Check sheet for the modelled part. Datum: model origin and axes. Units: mm. A direction names the side the tool comes from. Coordinates: 2 decimals unless noted, no trailing zeros. Order: outer loops, then holes, each group sorted by start corner. A loop starts at its lowest first (then second) coordinate and runs counter-clockwise, first axis right, second up. Notation, with made-up numbers: (-20.5, 29) -> (-1.5, 29) arc R30 cw to (-1.5, 68) -> close; hole circle Ø3 at (34.25, 34.25). An arc over 180 degrees is marked (long way). Put each result on its own line as item: value. Start each with the question number.
```python
from build123d import *

# Parameters (mm, degrees)
SKETCH1_W           = 98
SKETCH1_H           = 25
BOSS_EXTRUDE1_DEPTH = 10
CUT_EXTRUDE4_DEPTH  = 10
SKETCH4_W           = 25
SKETCH4_H           = 10
CUT_EXTRUDE6_DEPTH  = 5
SKETCH5_W           = 25
SKETCH5_H           = 10
CUT_EXTRUDE7_DEPTH  = 5
SKETCH6_W           = 5
SKETCH6_H           = 10
CUT_EXTRUDE8_DEPTH  = 5
SKETCH7_W           = 5
SKETCH7_H           = 10
CUT_EXTRUDE9_DEPTH  = 5
SKETCH8_W           = 88
SKETCH8_H           = 5
CUT_EXTRUDE10_DEPTH = 2


with BuildPart() as part:
    # Sketch1 → Boss-Extrude1 (new body)
    with BuildSketch(Plane(origin=(0, 0, 0), x_dir=(1, 0, 0), z_dir=(0, 1, 0))):
        Rectangle(SKETCH1_W, SKETCH1_H)
    extrude(amount=BOSS_EXTRUDE1_DEPTH)

    # Sketch2 → Cut-Extrude4 (cut)
    with BuildSketch(Plane(origin=(0, 10, 0), x_dir=(1, 0, 0), z_dir=(0, 1, 0))):
        Polygon((-2.5, 2.403992328), (-2.5, -7.5), (-34, -7.5), (-34, 7.5), (-2.5, 7.5), align=None)
        Polygon((2.5, 2.403992328), (2.5, 7.5), (34, 7.5), (34, -7.5), (2.5, -7.5), align=None)
    extrude(amount=-CUT_EXTRUDE4_DEPTH, mode=Mode.SUBTRACT)

    # Sketch4 → Cut-Extrude6 (cut)
    with BuildSketch(Plane.ZY.offset(49)):
        with Locations((0, 5)):
            Rectangle(SKETCH4_W, SKETCH4_H)
    extrude(amount=-CUT_EXTRUDE6_DEPTH, mode=Mode.SUBTRACT)

    # Sketch5 → Cut-Extrude7 (cut)
    with BuildSketch(Plane(origin=(49, 0, 0), x_dir=(0, 0, -1), z_dir=(1, 0, 0))):
        with Locations((0, 5)):
            Rectangle(SKETCH5_W, SKETCH5_H)
    extrude(amount=-CUT_EXTRUDE7_DEPTH, mode=Mode.SUBTRACT)

    # Sketch6 → Cut-Extrude8 (cut)
    with BuildSketch(Plane(origin=(44, 0, 0), x_dir=(0, 0, -1), z_dir=(1, 0, 0))):
        with Locations((0, 5)):
            Rectangle(SKETCH6_W, SKETCH6_H)
    extrude(amount=-CUT_EXTRUDE8_DEPTH, mode=Mode.SUBTRACT)

    # Sketch7 → Cut-Extrude9 (cut)
    with BuildSketch(Plane.ZY.offset(44)):
        with Locations((0, 5)):
            Rectangle(SKETCH7_W, SKETCH7_H)
    extrude(amount=-CUT_EXTRUDE9_DEPTH, mode=Mode.SUBTRACT)

    # Sketch8 → Cut-Extrude10 (cut)
    with BuildSketch(Plane(origin=(0, 0, -12.5), x_dir=(-1, 0, 0), z_dir=(0, 0, -1))):
        with Locations((0, 7.5)):
            Rectangle(SKETCH8_W, SKETCH8_H)
    extrude(amount=-CUT_EXTRUDE10_DEPTH, mode=Mode.SUBTRACT)


solid = part.part
```
1) Sectioned sample at C-C (x = 22). Record the boundary of the cut face in (y, z), plus the area to 3 significant figures.
2) Scan lines: line 1 along X through (y, z) = (8.75, -7); line 2 along X through (y, z) = (3.5, 1.5); line 3 along Z through (x, y) = (-29.5, 3). Record each from-to range of solid material in increasing order. Write a range as [from, to].
3) Access from +Z, -Z, +X, -X, +Y, -Y to the whole of each face (thin tool, end or side, straight path). Record for faces 3 (the flat face through (-39, 5, 0)), 4 (the flat face through (1, 5, -12)), 5 (the flat face through (42, 5, -2.5)), 6 (the flat face through (-1, 0, 0)), 7 (the flat face through (34, 5, 0)).
4) Sectioned sample at D-D (z = -0.5). Record the boundary of the cut face in (x, y).
5) Sectioned sample at A-A (z = 4). Record the boundary of the cut face in (x, y).
6) Gauge pin test, flat ends, axial feed: pin 1 (1 mm diameter, centred on x = -7.5, z = -11.5, fed in from +Y); pin 2 (12 mm diameter, centred on x = 11.5, z = 5, fed in from +Y); pin 3 (2.5 mm diameter, centred on y = 6.5, z = -1, fed in from +X); pin 4 (8 mm diameter, centred on x = 25.5, z = 0.5, fed in from +Y). Record the tip position at first contact, or that the pin passes through.
7) Sectioned sample at B-B (y = 7.75). Record the boundary of the cut face in (x, z), plus the area to 3 significant figures.
8) Mould release check, pull along Z, two halves, no side actions. Record for faces 1 (the flat face through (-44, 5, 7)), 2 (the flat face through (-2.5, 5, 0)): +Z half, -Z half, draft (parallel to the pull), parting line (faces both ways), or undercut.
Entries:
1. outline: (0, -12.5) -> (5, -12.5) -> (5, -10.5) -> (10, -10.5) -> (10, -7.5) -> (0, -7.5) -> close; (0, 7.5) -> (10, 7.5) -> (10, 12.5) -> (0, 12.5) -> close
1. area: 90.0 mm2
2. line 1: x = [-44, -34], [-2.5, 2.5], [34, 44]
2. line 2: x = [-39, -34], [-2.5, 2.5], [34, 39]
2. line 3: z = [-12.5, -7.5], [7.5, 12.5]
3. face 3: -X, +Y, -Y
3. face 4: -Z, +X, -X, +Y
3. face 5: +X, +Y, -Y
3. face 6: +Z, -Z, +X, -X, -Y
3. face 7: +Y, -Y
4. outline: (-39, 0) -> (-34, 0) -> (-34, 10) -> (-39, 10) -> close; (-2.5, 0) -> (2.5, 0) -> (2.5, 10) -> (-2.5, 10) -> close; (34, 0) -> (39, 0) -> (39, 10) -> (34, 10) -> close
5. outline: (-44, 0) -> (-34, 0) -> (-34, 10) -> (-44, 10) -> close; (-2.5, 0) -> (2.5, 0) -> (2.5, 10) -> (-2.5, 10) -> close; (34, 0) -> (44, 0) -> (44, 10) -> (34, 10) -> close
6. pin 1: stops at y = 5
6. pin 2: stops at y = 10
6. pin 3: stops at x = 39
6. pin 4: passes through
7. outline: (-44, -10.5) -> (44, -10.5) -> (44, -2.5) -> (39, -2.5) -> (39, 2.5) -> (44, 2.5) -> (44, 12.5) -> (-44, 12.5) -> (-44, 2.5) -> (-39, 2.5) -> (-39, -2.5) -> (-44, -2.5) -> close; hole (-34, -7.5) -> (-2.5, -7.5) -> (-2.5, 7.5) -> (-34, 7.5) -> close; hole (2.5, -7.5) -> (34, -7.5) -> (34, 7.5) -> (2.5, 7.5) -> close
7. area: 1,030 mm2
8. face 1: draft
8. face 2: undercut
